Could you check a few things on this drawing? It's one solid part, dimensions in mm from its lowest x, y, z. Give positions to 0.01 mm unless a question says otherwise; leave off trailing zeros. Order: outer loops, then holes, each group sorted by start corner. A loop starts at its lowest first (then second) coordinate and runs counter-clockwise, first axis right, second up. Notation, with made-up numbers: (11.5, -0.75) -> (42.5, -0.75) arc R22 ccw to (42.5, 21.25) -> close; hole circle Ø9 at (68, 31.25). An arc over 180 degrees is marked (long way). Answer as a JSON object with one key per item and string values.
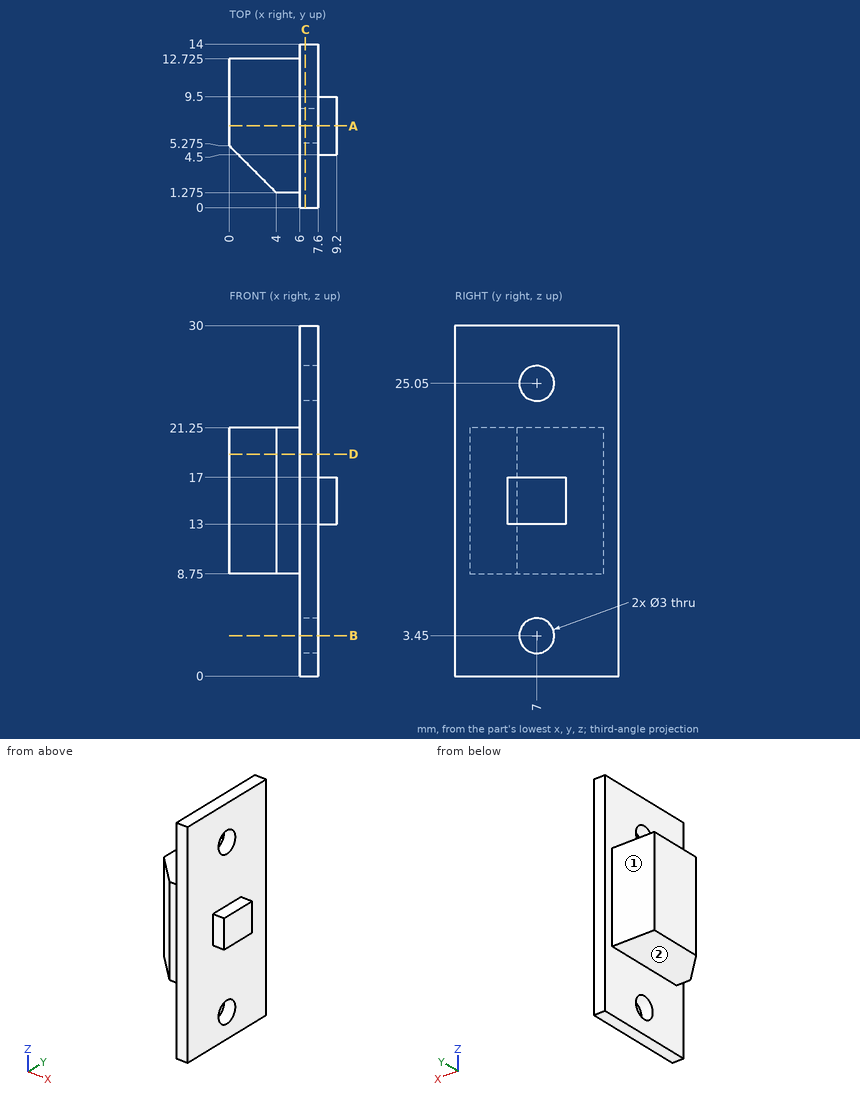
1. Will these pins go through, and if not, where does the flat tip stop? pin 1 Ø4 at (y, z) = (7, 3.45) entering from +X; pin 2 Ø0.5 at (x, z) = (8.5, 15.5) entering from -Y; pin 3 Ø1.8 at (x, y) = (2.5, 8.5) entering from +Z; pin 4 Ø3 at (x, y) = (8, 10) entering from -Z.
Worked answers:
{"pin 1": "x = 7.6", "pin 2": "y = 4.5", "pin 3": "z = 21.25", "pin 4": "z = 0"}
2. Please list where these lines run through material, in increasing order: L1, parallel to Z at x = 6.8, y = 7; L2, parallel to X at y = 6.5, z = 10.75; L3, parallel to X at y = 4.75, z = 26.
Worked answers:
{"L1": "0 to 1.95, 4.95 to 23.55, 26.55 to 30", "L2": "0 to 7.6", "L3": "6 to 7.6"}
3. If we section it at D-D on z = 19: Please give me the cut outline in (x, y) (3 decimals), then the cut area to 3 significant figures.
Worked answers:
{"outline": "(0, 5.275) -> (4, 1.275) -> (6, 1.275) -> (6, 0) -> (7.6, 0) -> (7.6, 14) -> (6, 14) -> (6, 12.725) -> (0, 12.725) -> close", "area": "83.1 mm²"}
4. If we mould it in two halves opening along Y, with no side actions, what happens to the marked faces 1 and 2? For each: +Y half, -Y half, draft (parallel to the pull), parting line (faces both ways), or undercut.
Worked answers:
{"face 1": "+Y half", "face 2": "draft"}
5. If we section it at A-A on y = 7: Please give me the cut outline in (x, z).
Worked answers:
{"outline": "(0, 8.75) -> (6, 8.75) -> (6, 4.95) -> (7.6, 4.95) -> (7.6, 13) -> (9.2, 13) -> (9.2, 17) -> (7.6, 17) -> (7.6, 23.55) -> (6, 23.55) -> (6, 21.25) -> (0, 21.25) -> close; (6, 0) -> (7.6, 0) -> (7.6, 1.95) -> (6, 1.95) -> close; (6, 26.55) -> (7.6, 26.55) -> (7.6, 30) -> (6, 30) -> close"}
6. If we section it at C-C on x = 6.5: Please give me the cut outline in (y, z).
Worked answers:
{"outline": "(0, 0) -> (14, 0) -> (14, 30) -> (0, 30) -> close; hole circle Ø3 at (7, 3.45); hole circle Ø3 at (7, 25.05)"}
7. If we section it at B-B on z = 3.45: Please give me the cut outline in (x, y).
Worked answers:
{"outline": "(6, 0) -> (7.6, 0) -> (7.6, 5.5) -> (6, 5.5) -> close; (6, 8.5) -> (7.6, 8.5) -> (7.6, 14) -> (6, 14) -> close"}
